Verification items for the finished model (mm, model axes). Face numbers are marked on the shaded views. A direction names the side the tool comes from. Give positions to 0.01 mm unless a question says otherwise; leave off trailing zeros. Loops run counter-clockwise (first coordinate to the right, second up) from the corner with the lowest first, then second, coordinate; pieces in that order, holes last. Notation, with made-up numbers: (-7.75, 23.5) -> (46.25, 23.5) arc R31 cw to (46.25, 58.5) -> close; hole circle Ø1 at (74, 15.25). An arc over 180 degrees is marked (long way). Answer in a Markdown table with one row per item. Add a question column.
Q1. Section check C-C on x = -163. Enter the section's corners in (y, z), and give its area (3 significant figures).
Q2. Material ranges on probe 1 along X at (y, z) = (27, -13.5); probe 2 along X at (y, z) = (-51, -17); probe 3 along X at (y, z) = (-26, 38), recorded low to high.
Q3. Set-up check for the marked faces 4, 5 and 6: record each of +Z, -Z, +X, -X, +Y, -Y from which the full face is reachable in a straight line by a thin tool's end or side.
Q4. Release check for a two-part mould opening along X. For the marked faces 1, 2 and 3 record: pulls with the +X half, pulls with the -X half, needs draft (parallel to the pull), parting line crosses it, or undercut.
Q5. Gauge pin test, flat ends, axial feed: P1, Ø13, axis at y = 146.5, z = -7.5, coming from the +X side; P2, Ø1, axis at x = -210, z = -0.5, coming from the +Y side; P3, Ø8, axis at x = -43.5, y = -19, coming from the -Z side. Record the tip position at first contact, or that the pin passes through.
Q6. Section check B-B on y = 27. Enter the section's corners in (x, z), and give its area (3 significant figures).
Q7. Section check A-A on x = 21. Enter the section's corners in (y, z), and give its area (3 significant figures).
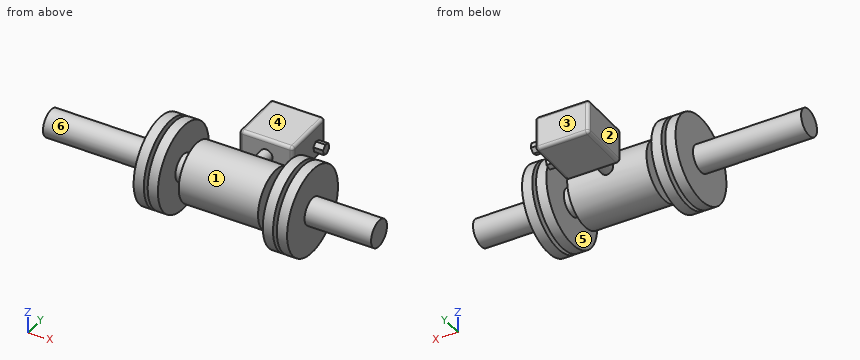
```python
from build123d import *

# Parameters (mm, degrees)
SKETCH_4_R      = 10
EXTRUDE_3_DEPTH = 165.5
SKETCH_5_W      = 84
SKETCH_5_H      = 54
EXTRUDE_4_DEPTH = 85
FILLET_1_R      = 5
EXTRUDE_5_DEPTH = 15


with BuildPart() as part:
    # Sketch 3 → Revolve 2 (revolve)
    with BuildSketch(Plane(origin=(0, 0, 0), x_dir=(1, 0, 0), z_dir=(0, 1, 0))):
        Polygon((82, -67.5), (98, -67.5), (98, -33), (104, -33), (104, -67.5), (120, -67.5), (120, -21.15), (224, -21.15), (224, 0), (-289, 0), (-289, -21.15), (-120, -21.15), (-120, -67.5), (-104, -67.5), (-104, -33), (-98, -33), (-98, -67.5), (-82, -67.5), (-82, -21.15), (-62, -21.15), (-62, -46.15), (62, -46.15), (62, -21.15), (82, -21.15), align=None)
    revolve(axis=Axis((-117.293644386, 0, 0), (1, 0, 0)))

    # Sketch 4 → Extrude 3 (add)
    with BuildSketch(Plane(origin=(0, 0, 0), x_dir=(1, 0, 0), z_dir=(0, 1, 0))):
        with Locations(Location((0, 0, 0), (0, 0, 90))):
            Circle(SKETCH_4_R)
    extrude(amount=EXTRUDE_3_DEPTH)

    # Sketch 5 → Extrude 4 (add)
    with BuildSketch(Plane(origin=(0, 165.5, 0), x_dir=(-1, 0, 0), z_dir=(0, 1, 0))):
        Rectangle(SKETCH_5_W, SKETCH_5_H)
    extrude(amount=-EXTRUDE_4_DEPTH)

    # Fillet 1
    fillet_1_edges = [part.edges().sort_by_distance(p)[0] for p in [
        (42, 165.5, 0),
        (0, 165.5, -27),
        (-42, 165.5, 0),
        (0, 165.5, 27),
        (42, 80.5, 0),
        (42, 123, -27),
        (0, 80.5, 27),
        (42, 123, 27),
        (-42, 80.5, 0),
        (-42, 123, 27),
        (0, 80.5, -27),
        (-42, 123, -27),
    ]]
    fillet(fillet_1_edges, radius=FILLET_1_R)

    # Sketch 6 → Extrude 5 (add)
    with BuildSketch(Plane(origin=(42, 0, 0), x_dir=(0, 0, -1), z_dir=(1, 0, 0))):
        Polygon((4.321367474, 134.764410902), (12.792913111, 136.562441636), (15.471545637, 144.798030734), (9.678632526, 151.235589098), (1.207086889, 149.437558364), (-1.471545637, 141.201969266), align=None)
        Polygon((-1.471545637, 104.798030734), (4.321367474, 111.235589098), (12.792913111, 109.437558364), (15.471545637, 101.201969266), (9.678632526, 94.764410902), (1.207086889, 96.562441636), align=None)
    extrude(amount=EXTRUDE_5_DEPTH)


solid = part.part
```
Taken from the geometry:
| question | item | result |
|---|---|---|
| 1 | outline | circle Ø42.3 at (0, 0) |
| 1 | area | 1,410 mm² |
| 2 | probe 1 | x = -120 to -82, -62 to 62, 82 to 120 |
| 2 | probe 2 | x = -120 to -104, -98 to -82, 82 to 98, 104 to 120 |
| 2 | probe 3 | x = -120 to -104, -98 to -82, -62 to 62, 82 to 98, 104 to 120 |
| 3 | face 4 | +Z, +X, -X, +Y |
| 3 | face 5 | none |
| 3 | face 6 | -X |
| 4 | face 1 | undercut |
| 4 | face 2 | pulls with the -X half |
| 4 | face 3 | needs draft |
| 5 | P1 | stops at x = 57 |
| 5 | P2 | stops at y = 21.15 |
| 5 | P3 | stops at z = -43.64 |
| 6 | outline | (-120, -61.86) -> (-104, -61.86) -> (-104, -18.97) -> (-98, -18.97) -> (-98, -61.86) -> (-82, -61.86) -> (-82, 61.86) -> (-98, 61.86) -> (-98, 18.97) -> (-104, 18.97) -> (-104, 61.86) -> (-120, 61.86) -> close; (-62, -37.43) -> (62, -37.43) -> (62, 37.43) -> (-62, 37.43) -> close; (82, -61.86) -> (98, -61.86) -> (98, -18.97) -> (104, -18.97) -> (104, -61.86) -> (120, -61.86) -> (120, 61.86) -> (104, 61.86) -> (104, 18.97) -> (98, 18.97) -> (98, 61.86) -> (82, 61.86) -> close |
| 6 | area | 17,700 mm² |
| 7 | outline | circle Ø92.3 at (0, 0); (80.5, -22) arc R5 ccw to (85.5, -27) -> (160.5, -27) arc R5 ccw to (165.5, -22) -> (165.5, 22) arc R5 ccw to (160.5, 27) -> (85.5, 27) arc R5 ccw to (80.5, 22) -> close |
| 7 | area | 11,300 mm² |
